from build123d import *

# Parameters (mm, degrees)
F1_DEPTH = 25
F2_R     = 5
F3_R     = 9
F4_DEPTH = 25.001


with BuildPart() as f1:
    # F0 (on Front) → F1 (new body)
    with BuildSketch(Plane.XZ):
        Polygon((46.278606, 27.882919), (-53.721394, 27.882919), (-53.185202, -22.117081), (46.278606, -22.117081), align=None)
    extrude(amount=F1_DEPTH)

    # F2
    f2_edges = [f1.edges().sort_by_distance(p)[0] for p in [
        (-3.453298, 0, -22.117081),
        (-3.453298, -25, -22.117081),
        (46.278606, -25, 2.882919),
        (-3.721394, -25, 27.882919),
        (-53.453298, -25, 2.882919),
        (46.278606, -12.5, 27.882919),
        (-53.721394, -12.5, 27.882919),
        (-3.721394, 0, 27.882919),
        (46.278606, 0, 2.882919),
        (-53.453298, 0, 2.882919),
        (46.278606, -12.5, -22.117081),
    ]]
    fillet(f2_edges, radius=F2_R)

    # F3 (on Front) → F4 (cut, through all)
    with BuildSketch(Plane.XZ):
        with Locations((-35.826672, 12.018532)):
            Circle(F3_R)
        with Locations((-35.826672, -7.581468)):
            Circle(F3_R)
        with Locations((-4.226672, 12.018532)):
            Circle(F3_R)
        with Locations((-4.226672, -7.581468)):
            Circle(F3_R)
        with Locations((27.373328, 12.018532)):
            Circle(F3_R)
        with Locations((27.373328, -7.581468)):
            Circle(F3_R)
    extrude(amount=F4_DEPTH, mode=Mode.SUBTRACT)


solid = f1.part
Read the model definition and answer for the solid it produces. Units are mm, in the model's axes. A direction names the side the tool comes from. Round coordinates to 2 decimals unless told otherwise and drop trailing zeros. Loops run counter-clockwise (first coordinate to the right, second up) from the corner with the lowest first, then second, coordinate; pieces in that order, holes last.
Q1. Section A-A on x = 3 is taken. Write down the section's boundary in (y, z).
Q2. Consider probe 1 along X at (y, z) = (-12.25, 6.5); probe 2 along Z at (x, y) = (-38, -3.25); probe 3 along Z at (x, y) = (0, -6.25). Determine where each line is inside the solid, lowest interval first.
Q3. Section C-C on x = 15.5 is taken. Write down the section's boundary in (y, z), and give its area (3 significant figures).
Q4. Section D-D on z = 16 is taken. Give the number of separate pieces and of enclosed holes in the cut face, and give its area (3 significant figures).
Q5. Which of the six approach directions +Z, -Z, +X, -X, +Y, -Y give full straight-line access (tool end or side, diameter ignored) to faces 1 (the face through (-51.997, -1.504, 0.057)), 2 (the face through (44.85, -23.5, 3.16))?
Q6. Section B-B on y = -21.25 is taken. Write down the section's boundary in (x, z), and give its area (3 significant figures).
Output:
1. outline: (-25, -17.12) arc R5 ccw to (-20, -22.12) - (-5, -22.12) arc R5 ccw to (0, -17.12) - (0, -12.95) - (-25, -12.95) - close; (-25, -2.22) - (0, -2.22) - (0, 6.65) - (-25, 6.65) - close; (-25, 17.38) - (0, 17.38) - (0, 22.88) arc R5 ccw to (-5, 27.88) - (-20, 27.88) arc R5 ccw to (-25, 22.88) - close
2. probe 1: x = -53.49 to -42.94, -28.72 to -11.34, 2.88 to 20.26, 34.48 to 46.28
2. probe 2: z = -21.8 to -16.32, 1.15 to 3.28, 20.75 to 27.57
2. probe 3: z = -22.12 to -15.53, 0.36 to 4.07, 19.96 to 27.88
3. outline: (-25, -17.12) arc R5 ccw to (-20, -22.12) - (-5, -22.12) arc R5 ccw to (0, -17.12) - (0, 22.88) arc R5 ccw to (-5, 27.88) - (-20, 27.88) arc R5 ccw to (-25, 22.88) - close
3. area: 1,230 mm2
4. separate pieces: 4
4. enclosed holes: 0
4. area: 1,260 mm2
5. face 1: -Z, -X, +Y
5. face 2: +Z, -Z, +X, -Y
6. outline: (-53.51, 22.83) - (-53.03, -21.96) - (41.28, -21.96) arc R4.84 ccw to (46.12, -17.12) - (46.12, 22.88) arc R4.84 ccw to (41.28, 27.72) - (-48.67, 27.72) arc R4.84 ccw to start; hole circle Ø18 at (-35.83, -7.58); hole circle Ø18 at (-35.83, 12.02); hole circle Ø18 at (-4.23, -7.58); hole circle Ø18 at (-4.23, 12.02); hole circle Ø18 at (27.37, -7.58); hole circle Ø18 at (27.37, 12.02)
6. area: 3,400 mm2
